The model under review builds one solid part; all positions refer to its coordinate system, in mm. A direction names the side the tool comes from. Coordinates: 2 decimals unless noted, no trailing zeros. Write each loop counter-clockwise with the first axis right and the second up, starting at its lowest first coordinate (ties: lowest second). Pieces come first, ordered by that corner, then holes. Notation, with made-up numbers: (-26.75, -12.75) -> (31.25, -12.75) arc R22 cw to (31.25, 3.25) -> close; hole circle Ø8 at (53.25, 20). An arc over 180 degrees is marked (long way). Write each question's results on one line, items separated by ' | '.
```python
from build123d import *

# Parameters (mm, degrees)
SKETCH1_R           = 3.5
BOSS_EXTRUDE1_DEPTH = 2
SKETCH2_R           = 1.5
BOSS_EXTRUDE2_DEPTH = 7
SKETCH5_OUTSIDE_W   = 11.676
SKETCH5_OUTSIDE_H   = 11.676
CUT_EXTRUDE1_DEPTH  = 7
BOSS_EXTRUDE4_DEPTH = 5
CHAMFER3_SIZE       = 0.3
CHAMFER3_SIZE2      = 1.701384546
CHAMFER4_SIZE       = 0.2
CHAMFER4_SIZE2      = 1.134256364
CUT_EXTRUDE2_DEPTH  = 3


with BuildPart() as part:
    # Sketch1 → Boss-Extrude1 (new body)
    with BuildSketch(Plane(origin=(0, 0, 0), x_dir=(1, 0, 0), z_dir=(0, 1, 0))):
        Circle(SKETCH1_R)
    extrude(amount=BOSS_EXTRUDE1_DEPTH)

    # Sketch2 → Boss-Extrude2 (add)
    with BuildSketch(Plane(origin=(0, 2, 0), x_dir=(1, 0, 0), z_dir=(0, 1, 0))):
        Circle(SKETCH2_R)
    extrude(amount=BOSS_EXTRUDE2_DEPTH)

    # Sketch5 outside → Cut-Extrude1 (cut)
    with BuildSketch(Plane(origin=(0, 2, 0), x_dir=(1, 0, 0), z_dir=(0, 1, 0))):
        Rectangle(SKETCH5_OUTSIDE_W, SKETCH5_OUTSIDE_H)
        with BuildLine():
            Line((-2.228687609, 2.698694414), (2.698694414, -2.228687609))
            ThreePointArc((2.698694414, -2.228687609), (2.111573719, -2.791282219), (1.41047572, -3.203210615))
            Line((1.41047572, -3.203210615), (-3.203210615, 1.41047572))
            ThreePointArc((-3.203210615, 1.41047572), (-2.791282219, 2.111573719), (-2.228687609, 2.698694414))
        make_face(mode=Mode.SUBTRACT)
    extrude(amount=CUT_EXTRUDE1_DEPTH, mode=Mode.SUBTRACT)

    # Sketch4 → Boss-Extrude4 (add)
    with BuildSketch(Plane(origin=(0, 2, 0), x_dir=(1, 0, 0), z_dir=(0, 1, 0))):
        with BuildLine():
            Line((0, 2.3), (0, 3.5))
            ThreePointArc((0, 3.5), (2.474873734, 2.474873734), (3.5, 0))
            Line((3.5, 0), (2.3, 0))
            ThreePointArc((2.3, 0), (1.626345597, 1.626345597), (0, 2.3))
        make_face()
    extrude(amount=BOSS_EXTRUDE4_DEPTH)

    # Chamfer3
    chamfer3_edges = [part.edges().sort_by_distance(p)[0] for p in [
        (0.235003403, 2, -0.235003403),
    ]]
    chamfer3_side = [part.faces().sort_by_distance(p)[0] for p in [
        (-2.404873734, 2, 2.404873734),
    ]]
    chamfer(chamfer3_edges, length=CHAMFER3_SIZE, length2=CHAMFER3_SIZE2, reference=chamfer3_side[0])

    # Chamfer4
    chamfer4_edges = [part.edges().sort_by_distance(p)[0] for p in [
        (-0.896367447, 2, 0.896367447),
    ]]
    chamfer4_side = [part.faces().sort_by_distance(p)[0] for p in [
        (-0.704284953, 2, -1.435537374),
    ]]
    chamfer(chamfer4_edges, length=CHAMFER4_SIZE, length2=CHAMFER4_SIZE2, reference=chamfer4_side[0])

    # Sketch6 → Cut-Extrude2 (cut, through all)
    with BuildSketch(Plane(origin=(0, 2, 0), x_dir=(1, 0, 0), z_dir=(0, 1, 0))):
        with BuildLine():
            Line((-2.5, 0), (-2.5, 2.449489743))
            ThreePointArc((-2.5, 2.449489743), (-2.474873734, -2.474873734), (2.449489743, -2.5))
            Line((2.449489743, -2.5), (0, -2.5))
            ThreePointArc((0, -2.5), (-1.767766953, -1.767766953), (-2.5, 0))
        make_face()
    extrude(amount=-CUT_EXTRUDE2_DEPTH, mode=Mode.SUBTRACT)


solid = part.part
```
Q1. Clearance check with flat-ended pins moving along their axes: P1, Ø1, axis at y = 3.5, z = -3, coming from the -X side; P2, Ø1.5, axis at x = -1.5, z = -0.5, coming from the -Y side; P3, Ø1.8, axis at x = 1.5, z = -1.5, coming from the +Y side; P4, Ø3, axis at x = 1.5, y = 6, coming from the +Z side. State where each tip first meets the part, or that it passes through.
Solution:
P1: x = 0 | P2: y = 0 | P3: y = 7 | P4: z = 1.5
Q2. Draft analysis for pull direction X (two halves, no side actions). For faces 4 (the flat face through (2, 7, -2)), 5 (the cylindrical face through (1.64, 4.46, -1.61)), 6 (the cylindrical face through (-1.748, 1.014, 1.787)), state which applies: pulls with the +X half, pulls with the -X half, needs draft (parallel to the pull), parting line crosses it, or undercut.
Solution:
face 4: needs draft | face 5: undercut | face 6: pulls with the -X half
Q3. Machinability: for faces 1 (the flat face through (3, 4, 0)), 2 (the flat face through (0.33, 2.86, -0.35)), 3 (the cylindrical face through (0.456, 5.451, 1.429)), which of the approach directions +Z, -Z, +X, -X, +Y, -Y give a long, thin tool a straight path to every point of the face, cutting with its end or side? Answer none if there is none.
Solution:
face 1: +Z, +X, +Y | face 2: +Y | face 3: +Z, +Y
Q4. Add section A-A (y = 3.25). Write out the cut boundary in (x, z), plus the area to 3 significant figures.
Solution:
outline: (-1.46, 0.33) arc R1.5 ccw to (-0.73, -1.31) -> (1.31, 0.73) arc R1.5 ccw to (-0.33, 1.46) -> close; (0, -3.5) arc R3.5 ccw to (3.5, 0) -> (2.3, 0) arc R2.3 cw to (0, -2.3) -> close | area: 9.97 mm²
Q5. Add section D-D (x = 3.05). Write out the cut boundary in (y, z), plus the area to 3 significant figures.
Solution:
outline: (0, -1.72) -> (7, -1.72) -> (7, 0) -> (2, 0) -> (2, 1.72) -> (0, 1.72) -> close | area: 15.5 mm²
Q6. Add section B-B (x = -1). Write out the cut boundary in (y, z), plus the area to 3 significant figures.
Solution:
outline: (0, -3.35) -> (2, -3.35) -> (2, -1.12) -> (9, -1.12) -> (9, 0.79) -> (3.13, 0.79) -> (2, 1.08) -> (2, 2.29) -> (0, 2.29) -> close | area: 24.8 mm²
Q7. Add section C-C (z = -2). Write out the cut boundary in (x, y), plus the area to 3 significant figures.
Solution:
outline: (-2.5, 0) -> (2.87, 0) -> (2.87, 7) -> (1.14, 7) -> (1.14, 2) -> (-2.5, 2) -> close | area: 19.4 mm²
Q8. For line 1 (Y direction, x = -0.05, z = 2); line 2 (Y direction, x = 0.5, z = -2.5); line 3 (Z direction, x = 0.65, y = 6.5), list the stretches that pass through material, from the lowest coordinate up. Write a range as from..to.
Solution:
line 1: 0..2 | line 2: 0..7 | line 3: -3.44..-2.21, 0.18..1.35
